Autodesk Inventor part; units mm, degrees
ref_plane "YZ Plane" through (0, 0, 0) normal (1, 0, 0) x (0, 1, 0)
ref_plane "XZ Plane" through (0, 0, 0) normal (0, 1, 0) x (-1, 0, 0)
ref_plane "XY Plane" through (0, 0, 0) normal (0, 0, 1) x (1, 0, 0)
sketch "スケッチ1" plane through (0, 0, 0) normal (0, 1, 0) x (-1, 0, 0)
  line L0 (0, 0) -> (12, 0)
  line L1 (12, 0) -> (12, -12)
  line L2 (12, -12) -> (0, -12)
  line L3 (0, -12) -> (0, 0)
  dimension "d0" = 12
  dimension "d1" = 12
extrude "押し出し1" add sketch "スケッチ1" along normal blind 10
sketch "スケッチ2" plane through (0, 10, 0) normal (0, 1, 0) x (1, 0, 0)
  line L0 (-12, 0) -> (0, 0)
  line L1 (-6, 0) -> (-6, 12)
  line L2 (0, 12) -> (-12, 12)
  line L3 (-12, 12) -> (-12, 0)
  line L4 (-12, 6) -> (0, 6)
  circle A0 centre (-6, 6) radius 5.5
  dimension "d4" = 11
extrude "押し出し2" add sketch "スケッチ2" along normal blind 39 contours A0 L4 L1 | L1 L4 A0 | A0 L1 L4 | L1 A0 L4
sketch "スケッチ3" plane through (-6, 49, -6) normal (0, 1, 0) x (1, 0, 0)
  line L0 (-6, 6) -> (-6, -6)
  line L1 (6, -6) -> (6, 6)
  line L2 (-6, 6) -> (6, 6)
  line L3 (6, 6) -> (6, -6)
  line L4 (6, -6) -> (-6, -6)
  line L5 (-6, -6) -> (-6, 6)
extrude "押し出し3" add sketch "スケッチ3" along normal blind 13
fillet "フィレット1" radius 2 8 edges at (0, 55.5, 0) (0, 5, 0) (0, 5, -12) (0, 55.5, -12) (-12, 55.5, 0) (-12, 5, 0) (-12, 5, -12) (-12, 55.5, -12)
sketch "スケッチ4" plane through (-6, 62, -6) normal (0, 1, 0) x (1, 0, 0)
  circle A0 centre (0, 0) radius 4
  point P0 (6, -6)
  dimension "d10" = 8
extrude "押し出し4" add sketch "スケッチ4" along normal blind 8
sketch "スケッチ5" plane through (-6, 70, -6) normal (0, 1, 0) x (1, 0, 0)
  circle A0 centre (0, 0) radius 2
  point P0 (6, -6)
  dimension "d13" = 4
extrude "押し出し5" cut sketch "スケッチ5" against normal blind 15
properties part number "summer_cilinder"
Could you check a few things on this model? Use its own coordinates, in mm. A direction names the side the tool comes from. Coordinates: 2 decimals unless noted, no trailing zeros. Order: outer loops, then holes, each group sorted by start corner. A loop starts at its lowest first (then second) coordinate and runs counter-clockwise, first axis right, second up.
Q1. Suppose I cut it at C-C on z = -6. Please give me the cut outline in (x, y).
Q2. Which directions (+Z, -Z, +X, -X, +Y, -Y) give clear straight access to the entire face, cutting with the end or side of a thin tool? Please do faces 1 (the flat face through (-6, 5, -12)), 2 (the flat face through (-6, 55, -6)).
Q3. Suppose I cut it at D-D on y = 45.5. Please give me the cut outline in (x, z).
Q4. Please list where these lines run through material, in increasing order: L1, parallel to Z at x = -6, y = 59; L2, parallel to Y at x = -8.5, z = -1.
Q5. Thinking about a two-plate mould opening in Y: for faces 3 (the flat face through (0, 55, -6)), 4 (the flat face through (-8, 70, -5)), 5 (the flat face through (-9, 49, -1)), which applies, released by +Y, released by -Y, zero draft, split by the parting line, or undercut?
Q6. Suppose I cut it at B-B on x = -6. Please give me the cut outline in (y, z).
Q7. Will these pins go through, and if not, where does the flat tip stop? pin 1 (6 mm diameter, centred on x = -6.5, y = 44, fed in from +Z); pin 2 (3.5 mm diameter, centred on x = -8, z = -4, fed in from -Y); pin 3 (1 mm diameter, centred on y = 48, z = -3, fed in from +X); pin 4 (4 mm diameter, centred on y = 33, z = -3, fed in from +X).
Q8. Suppose I cut it at A-A on y = 60. Please give me the cut outline in (x, z), and give its area (3 significant figures).
Answer:
1. outline: (-12, 0) - (0, 0) - (0, 10) - (-0.5, 10) - (-0.5, 49) - (0, 49) - (0, 62) - (-2, 62) - (-2, 70) - (-4, 70) - (-4, 55) - (-8, 55) - (-8, 70) - (-10, 70) - (-10, 62) - (-12, 62) - (-12, 49) - (-11.5, 49) - (-11.5, 10) - (-12, 10) - close
2. face 1: -Z, +X, -X, +Y, -Y
2. face 2: +Y
3. outline: circle Ø11 at (-6, -6)
4. L1: z = -12 to -8, -4 to 0
4. L2: y = 0 to 10, 49 to 62
5. face 3: zero draft
5. face 4: released by +Y
5. face 5: undercut
6. outline: (0, -12) - (10, -12) - (10, -11.5) - (49, -11.5) - (49, -12) - (62, -12) - (62, -10) - (70, -10) - (70, -8) - (55, -8) - (55, -4) - (70, -4) - (70, -2) - (62, -2) - (62, 0) - (49, 0) - (49, -0.5) - (10, -0.5) - (10, 0) - (0, 0) - close
7. pin 1: stops at z = -0.5
7. pin 2: stops at y = 0
7. pin 3: stops at x = -1.1
7. pin 4: stops at x = -0.59
8. outline: (-12, -10) arc R2 ccw to (-10, -12) - (-2, -12) arc R2 ccw to (0, -10) - (0, -2) arc R2 ccw to (-2, 0) - (-10, 0) arc R2 ccw to (-12, -2) - close; hole circle Ø4 at (-6, -6)
8. area: 128 mm2
